For this review, use the dimensioned drawing (mm, ordinates from the lowest corner) and the shaded views. Give positions to 0.01 mm unless a question says otherwise; leave off trailing zeros. Write each loop counter-clockwise with the first axis right and the second up, starting at its lowest first coordinate (ties: lowest second). Pieces come first, ordered by that corner, then holes. Notation, with made-up numbers: M 5.25,15.5 L 42.25,15.5 A37 ccw 42.25,52.5 Z; hole C 39,65 d7. An arc over 180 degrees is marked long. Use a Markdown table: item, result. Add a question column.
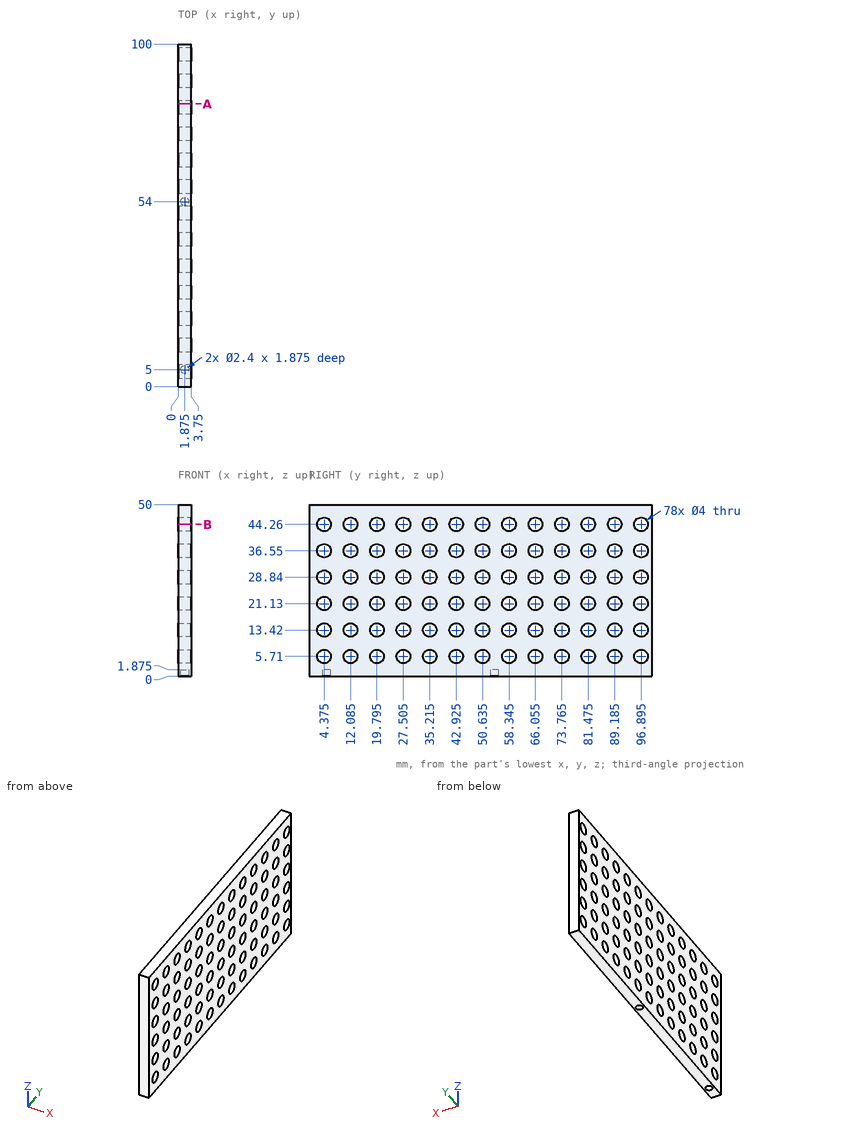
(1) Add section A-A on y = 82.5. Give the boundary of the cut face in (x, z).
(2) Add section B-B on z = 44.26. Give the number of separate pieces and of enclosed holes in the cut face, then the cut area to 3 significant figures.
(3) Wall thickness on L1, parallel to Z at x = 1.65, y = 53 (3 decimals): over which ranges is the line inside the solid? List them lowest first.
From the geometry:
| question | item | result |
|---|---|---|
| 1 | outline | M 0,0 L 3.75,0 L 3.75,3.99 L 0,3.99 Z; M 0,7.43 L 3.75,7.43 L 3.75,11.7 L 0,11.7 Z; M 0,15.14 L 3.75,15.14 L 3.75,19.41 L 0,19.41 Z; M 0,22.85 L 3.75,22.85 L 3.75,27.12 L 0,27.12 Z; M 0,30.56 L 3.75,30.56 L 3.75,34.83 L 0,34.83 Z; M 0,38.27 L 3.75,38.27 L 3.75,42.54 L 0,42.54 Z; M 0,45.98 L 3.75,45.98 L 3.75,50 L 0,50 Z |
| 2 | separate pieces | 14 |
| 2 | enclosed holes | 0 |
| 2 | area | 180 mm^2 |
| 3 | L1 | z = 1.875 to 50 |
